Source: three-view drawing plus pictorial views. Frame: mm from the lowest corner of the part. A direction names the side the tool comes from. Give positions to 0.01 mm unless a question says otherwise; leave off trailing zeros. Loops run counter-clockwise (first coordinate to the right, second up) from the corner with the lowest first, then second, coordinate; pieces in that order, holes last.
1. Section B-B, the plane z = 2. Output: boundary loops of the cut face in (x, y).
2. First-contact query: P1, Ø3, axis at x = 33, y = 5, coming from the -Z side. Flat tip, straight axial feed; report the tip coordinate or a pass-through.
3. Access query for the marked faces 5 and 6. Directions: +Z, -Z, +X, -X, +Y, -Y. A direction counts if a zero-diameter tool reaches every point of the face in a straight line with its end or side. Return the directions, or none.
4. Draft query along Y for the marked faces 1, 2, 3 and 4. Return one class per face: +Y half, -Y half, draft (parallel to the pull), parting line (faces both ways), or undercut.
5. Section D-D, the plane x = 23. Output: boundary loops of the cut face in (y, z) (1 decimal), then the cut area to 3 significant figures.
6. Section A-A, the plane y = 24.05. Output: boundary loops of the cut face in (x, z) (1 decimal).
7. Section C-C, the plane x = 5.5. Output: boundary loops of the cut face in (y, z), then the cut area to 3 significant figures.
8. Material intervals for line 1 along X through (y, z) = (36.5, 8.5) (1 decimal); line 2 along Y through (x, z) = (22.5, 11); line 3 along Y through (x, z) = (38.5, 3), sorted ascending.
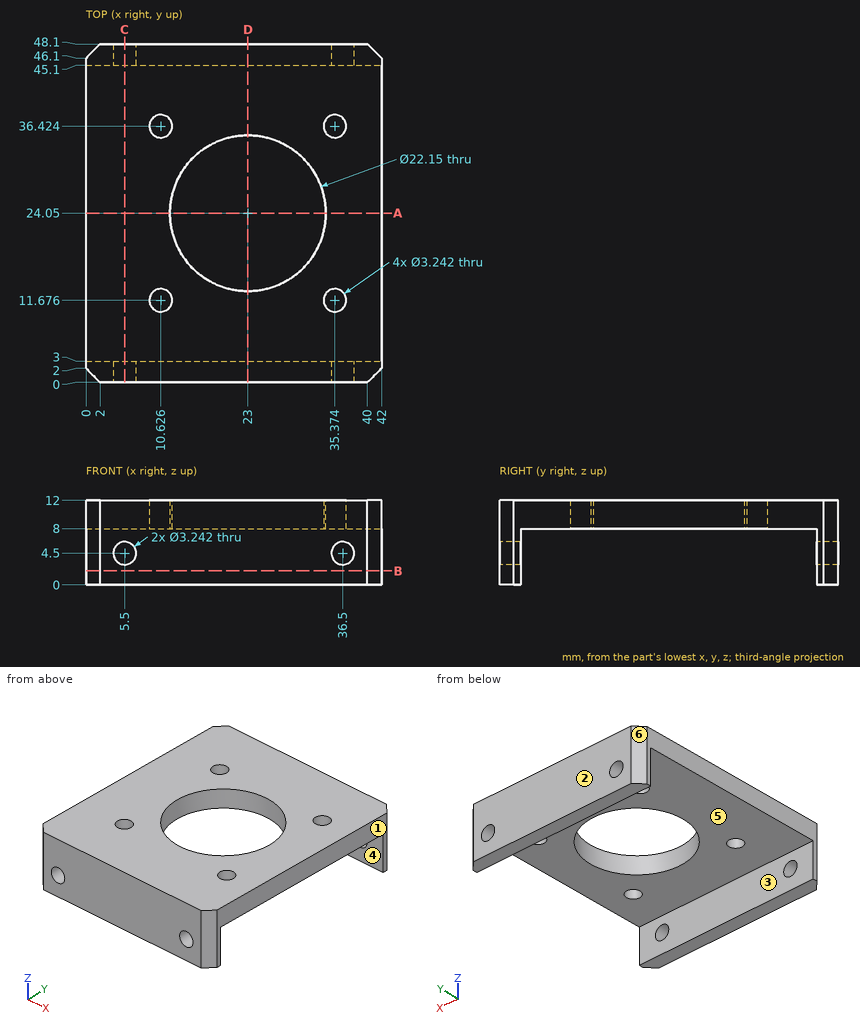
Answers below:
1. outline: (0, 2) - (2, 0) - (40, 0) - (42, 2) - (42, 3) - (0, 3) - close; (0, 45.1) - (42, 45.1) - (42, 46.1) - (40, 48.1) - (2, 48.1) - (0, 46.1) - close
2. P1: stops at z = 8
3. face 5: -Z, +X, -X
3. face 6: +Z, -Z, -X, +Y
4. face 1: draft
4. face 2: +Y half
4. face 3: undercut
4. face 4: undercut
5. outline: (0, 0) - (3, 0) - (3, 8) - (13, 8) - (13, 12) - (0, 12) - close; (35.1, 8) - (45.1, 8) - (45.1, 0) - (48.1, 0) - (48.1, 12) - (35.1, 12) - close
5. area: 152 mm2
6. outline: (0, 8) - (11.9, 8) - (11.9, 12) - (0, 12) - close; (34.1, 8) - (42, 8) - (42, 12) - (34.1, 12) - close
7. outline: (0, 0) - (3, 0) - (3, 2.88) - (0, 2.88) - close; (0, 6.12) - (3, 6.12) - (3, 8) - (45.1, 8) - (45.1, 6.12) - (48.1, 6.12) - (48.1, 12) - (0, 12) - close; (45.1, 0) - (48.1, 0) - (48.1, 2.88) - (45.1, 2.88) - close
7. area: 221 mm2
8. line 1: x = 0 to 9, 12.2 to 33.8, 37 to 42
8. line 2: y = 0 to 12.99, 35.11 to 48.1
8. line 3: y = 0 to 3, 45.1 to 48.1
